For this review, take the finished solid that the model builds, in its own axes (mm). A direction names the side the tool comes from. Round coordinates to 2 decimals unless told otherwise and drop trailing zeros. Order: outer loops, then holes, each group sorted by start corner. A loop starts at its lowest first (then second) coordinate and runs counter-clockwise, first axis right, second up. Notation, with made-up numbers: (11.5, 33) - (28.5, 33) arc R19 cw to (28.5, 51) - close; hole circle Ø2 at (60, 30.25). An arc over 180 degrees is marked (long way). Write each question's results on one line, items separated by ' | '. Start each with the question number.
(1) For faces 5 (the flat face through (-31, 47.5, 30)), 6 (the flat face through (1, 0, -25)), 7 (the cylindrical face through (-2.46, 1.08, -4.88)), list the 3-axis set-ups (+Z, -Z, +X, -X, +Y, -Y) from which the entire face can be reached by the end or side of a thin tool; tool diameter is ignored.
(2) For L1, parallel to X at y = 14, z = 16; L2, parallel to X at y = 35, z = 48; L3, parallel to X at y = 13, z = -8.5, list the stretches that pass through material, from the lowest coordinate up. Write a range as from..to.
(3) Insertion check: pin 1 Ø1.5 at (x, y) = (2, -6.5) entering from +Z; pin 2 Ø0.9 at (x, z) = (1, 22.5) entering from -Y; pin 3 Ø1.5 at (x, y) = (-31, 38.5) entering from -Z. Each pin has a flat end and moves straight along its axis. Give the tip position at first contact, or say it passes through.
(4) Draft analysis for pull direction Z (two halves, no side actions). For faces 1 (the cylindrical face through (-14.86, 4.88, 37.18)), 2 (the cylindrical face through (-27.46, 1.08, -4.88)), 3 (the flat face through (-31, -12.5, 12)), 4 (the flat face through (-31, -5, 50)), state which applies: pulls with the +Z half, pulls with the -Z half, needs draft (parallel to the pull), parting line crosses it, or undercut.
(5) Take a section at B-B, the plane y = 0. Give the boundary of the cut face in (x, z).
(6) Take a section at C-C, the plane z = -8. Give the boundary of the cut face in (x, y), plus the area to 3 significant figures.
(7) Take a section at D-D, the plane x = -39.5. Give the boundary of the cut face in (y, z).
(8) Take a section at A-A, the plane z = 36. Give the boundary of the cut face in (x, y), plus the area to 3 significant figures.
```python
from build123d import *

# Parameters (mm, degrees)
F1_DEPTH  = 3
F2_R      = 5
F3_DEPTH  = 5
F4_R      = 37.5
F5_DEPTH  = 20
F6_R      = 5
F7_DEPTH  = 5
F9_DEPTH  = 3
F10_W     = 90
F10_H     = 90
F11_DEPTH = 5


with BuildPart() as f1:
    # F0 (on Right) → F1 (new body)
    with BuildSketch(Plane.YZ):
        Polygon((-12.5, 50), (-12.5, -25), (12.5, -25), (12.5, 10), (47.5, 10), (47.5, 50), align=None)
    extrude(amount=F1_DEPTH)

    # F2 (on face) → F3 (join)
    with BuildSketch(Plane(origin=(0, 0, 0), x_dir=(0, -1, 0), z_dir=(-1, 0, 0))):
        Circle(F2_R)
    extrude(amount=F3_DEPTH)

    # F4 (on face) → F5 (join)
    with BuildSketch(Plane(origin=(-5, 0, 0), x_dir=(0, -1, 0), z_dir=(-1, 0, 0))):
        Circle(F4_R)
    extrude(amount=F5_DEPTH)

    # F6 (on face) → F7 (join)
    with BuildSketch(Plane(origin=(-25, 0, 0), x_dir=(0, -1, 0), z_dir=(-1, 0, 0))):
        Circle(F6_R)
    extrude(amount=F7_DEPTH)

    # F8 (on face) → F9 (join)
    with BuildSketch(Plane(origin=(-30, 0, 0), x_dir=(0, -1, 0), z_dir=(-1, 0, 0))):
        Polygon((12.5, 50), (-47.5, 50), (-47.5, 10), (-12.5, 10), (-12.5, -25), (12.5, -25), align=None)
    extrude(amount=F9_DEPTH)

    # F10 (on face) → F11 (join)
    with BuildSketch(Plane.XY.offset(50)):
        with Locations((-15, 47.5)):
            Rectangle(F10_W, F10_H)
    extrude(amount=F11_DEPTH)


solid = f1.part
```
Results below:
1) face 5: -Z, +X, -X, +Y | face 6: -Z, +X, +Y, -Y | face 7: none
2) L1: x = -33..-30, -25..-5, 0..3 | L2: x = -33..-30, 0..3 | L3: x = -25..-5
3) pin 1: stops at z = 50 | pin 2: stops at y = -12.5 | pin 3: stops at z = 10
4) face 1: undercut | face 2: undercut | face 3: needs draft | face 4: pulls with the +Z half
5) outline: (-33, -25) - (-30, -25) - (-30, -5) - (-25, -5) - (-25, -37.5) - (-5, -37.5) - (-5, -5) - (0, -5) - (0, -25) - (3, -25) - (3, 50) - (0, 50) - (0, 5) - (-5, 5) - (-5, 37.5) - (-25, 37.5) - (-25, 5) - (-30, 5) - (-30, 50) - (-33, 50) - close
6) outline: (-33, -12.5) - (-30, -12.5) - (-30, 12.5) - (-33, 12.5) - close; (-25, -36.64) - (-5, -36.64) - (-5, 36.64) - (-25, 36.64) - close; (0, -12.5) - (3, -12.5) - (3, 12.5) - (0, 12.5) - close | area: 1,620 mm^2
7) outline: (2.5, 50) - (92.5, 50) - (92.5, 55) - (2.5, 55) - close
8) outline: (-33, -12.5) - (-30, -12.5) - (-30, 47.5) - (-33, 47.5) - close; (-25, -10.5) - (-5, -10.5) - (-5, 10.5) - (-25, 10.5) - close; (0, -12.5) - (3, -12.5) - (3, 47.5) - (0, 47.5) - close | area: 780 mm^2
